Work out the finished part from the listing and answer in its coordinate system (mm). Coordinates: 2 decimals unless noted, no trailing zeros. Order: outer loops, then holes, each group sorted by start corner. A loop starts at its lowest first (then second) coordinate and runs counter-clockwise, first axis right, second up. Notation, with made-up numbers: (19, -7.5) -> (31, -7.5) arc R8 cw to (31, -2.5) -> close; hole circle Ø9 at (-11.75, 2.5). An arc over 180 degrees is marked (long way). Use one line per item in the form item = value.
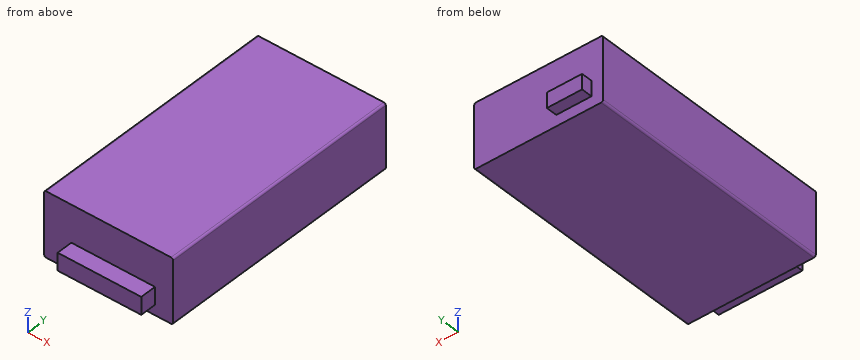
from build123d import *

# Parameters (mm, degrees)
F0_W     = 128
F0_H     = 64
F1_DEPTH = 248
F2_W     = 83
F2_H     = 17.327847
F3_DEPTH = 16
F4_W     = 35
F4_H     = 15
F5_DEPTH = 11
F6_R     = 2


with BuildPart() as f1:
    # F0 (on Front) → F1 (new body)
    with BuildSketch(Plane.XZ):
        with Locations((64, 32)):
            Rectangle(F0_W, F0_H)
    extrude(amount=F1_DEPTH)

    # F2 (on face) → F3 (join)
    with BuildSketch(Plane.XZ.offset(248)):
        with Locations((68.5, 18.663923)):
            Rectangle(F2_W, F2_H)
    extrude(amount=F3_DEPTH)

    # F4 (on face) → F5 (join)
    with BuildSketch(Plane(origin=(0, 0, 0), x_dir=(-1, 0, 0), z_dir=(0, 1, 0))):
        with Locations((-29, 18.5)):
            Rectangle(F4_W, F4_H)
    extrude(amount=F5_DEPTH)

    # F6
    f6_edges = [f1.edges().sort_by_distance(p)[0] for p in [
        (128, -124, 64),
        (128, -124, 0),
        (0, -124, 64),
        (0, -124, 0),
    ]]
    fillet(f6_edges, radius=F6_R)


solid = f1.part
(1) Section D-D on z = 47 is taken. Write down the section's boundary in (x, y), plus the area to 3 significant figures.
Data:
outline = (0, -248) -> (128, -248) -> (128, 0) -> (0, 0) -> close
area = 31,700 mm²
(2) Section B-B on z = 21.5 is taken. Write down the section's boundary in (x, y).
Data:
outline = (0, -248) -> (27, -248) -> (27, -264) -> (110, -264) -> (110, -248) -> (128, -248) -> (128, 0) -> (46.5, 0) -> (46.5, 11) -> (11.5, 11) -> (11.5, 0) -> (0, 0) -> close
(3) Section A-A on x = 23 is taken. Write down the section's boundary in (y, z), plus the area to 3 significant figures.
Data:
outline = (-248, 0) -> (0, 0) -> (0, 11) -> (11, 11) -> (11, 26) -> (0, 26) -> (0, 64) -> (-248, 64) -> close
area = 16,000 mm²
(4) Section C-C on x = 56 is taken. Write down the section's boundary in (y, z).
Data:
outline = (-264, 10) -> (-248, 10) -> (-248, 0) -> (0, 0) -> (0, 64) -> (-248, 64) -> (-248, 27.33) -> (-264, 27.33) -> close
(5) Straight lines are drawn through the part: line 1 along Y through (x, z) = (39, 8.5); line 2 along Y through (x, z) = (74, 12.5). For each, find the intervals that lie inside material, in ascending order.
Data:
line_1 = -248 to 0
line_2 = -264 to 0
(6) Each of these flat-tipped pins is pushed along its axis until it touches: P1, Ø19, axis at x = 72, z = 46.5, coming from the +Y side; P2, Ø13, axis at x = 63, y = -259, coming from the +Z side; P3, Ø9, axis at x = 25.5, y = 6.5, coming from the +Z side. Where does it stop, or does it pass through?
Data:
P1 = 0
P2 = 27.33
P3 = 26
